from build123d import *

# Parameters (mm, degrees)
F1_DEPTH      = 2.667
F1_DEPTH_BACK = 2.667
F2_W          = 95.25
F2_H          = 4.826
F3_DEPTH      = 9.525
F3_DEPTH_BACK = 9.525
F4_R          = 3.175
F4_R_2        = 7.14375
F5_DEPTH      = 3.556
F6_R          = 1.524
F7_DEPTH      = 10.16


with BuildPart() as f1:
    # F0 (on Right) → F1 (new body, two sides)
    with BuildSketch(Plane.YZ) as f1_sk:
        with BuildLine():
            Line((89.8299359697, 89.8299359697), (0, 0))
            Line((0, 0), (7.6651280605, 0))
            Line((7.6651280605, 0), (95.25, 0))
            Line((95.25, 0), (95.25, 87.5848719395))
            ThreePointArc((95.25, 87.5848719395), (93.2900198978, 90.5181894552), (89.8299359697, 89.8299359697))
        make_face()
        with BuildLine():
            ThreePointArc((38.3256403027, 12.7), (35.3923227869, 14.6599801022), (36.0805762724, 18.1200640303))
            Line((36.0805762724, 18.1200640303), (77.1299359697, 59.1694237276))
            ThreePointArc((77.1299359697, 59.1694237276), (80.5900198978, 59.8576772131), (82.55, 56.9243596973))
            Line((82.55, 56.9243596973), (82.55, 15.875))
            ThreePointArc((82.55, 15.875), (81.6200640303, 13.6299359697), (79.375, 12.7))
            Line((79.375, 12.7), (38.3256403027, 12.7))
        make_face(mode=Mode.SUBTRACT)
    extrude(amount=F1_DEPTH)
    extrude(f1_sk.sketch, amount=-F1_DEPTH_BACK)

    # F2 (on Right) → F3 (join, two sides)
    with BuildSketch(Plane.YZ) as f3_sk:
        with Locations((47.625, -2.413)):
            Rectangle(F2_W, F2_H)
    extrude(amount=F3_DEPTH)
    extrude(f3_sk.sketch, amount=-F3_DEPTH_BACK)

    # F4 (on face) → F5 (cut)
    with BuildSketch(Plane(origin=(0, 0, -4.826), x_dir=(1, 0, 0), z_dir=(0, 0, -1))):
        with Locations((0, -85.09)):
            Circle(F4_R)
        with Locations((0, -10.16)):
            Circle(F4_R)
        with Locations((0, -73.66)):
            Circle(F4_R_2)
        with Locations((0, -21.59)):
            Circle(F4_R_2)
    extrude(amount=-F5_DEPTH, mode=Mode.SUBTRACT)

    # F6 (on face) → F7 (cut)
    with BuildSketch(Plane(origin=(0, 0, -4.826), x_dir=(1, 0, 0), z_dir=(0, 0, -1))):
        with Locations((0, -85.09)):
            Circle(F6_R)
        with Locations((0, -10.16)):
            Circle(F6_R)
    extrude(amount=-F7_DEPTH, mode=Mode.SUBTRACT)


solid = f1.part
Input: part model. Units: mm. Frame: model coordinates. A direction names the side the tool comes from. Coordinates: 2 decimals unless noted, no trailing zeros. Loops run counter-clockwise (first coordinate to the right, second up) from the corner with the lowest first, then second, coordinate; pieces in that order, holes last.
Q1. Contact query for flat-ended pins moving along their axis: pin 1 (5 mm diameter, centred on x = 0, y = 10.16, fed in from -Z); pin 2 (12 mm diameter, centred on y = 12, z = 17, fed in from +X); pin 3 (1.5 mm diameter, centred on x = -1, z = 53, fed in from -Y). Output: stop coordinate, or through.
Q2. Cut plane A-A (z = 22). Output: boundary loops of the cut face in (x, y), then the cut area to 3 significant figures.
Q3. Draft query along Y for faces 6 (the face through (0.04, 56.32, 38.36)), 7 (the face through (0.037, 93.338, 90.498)), 8 (the face through (0, 82.55, 37)), 9 (the face through (-6, 47, 0)). Return one class per face: +Y half, -Y half, draft (parallel to the pull), parting line (faces both ways), or undercut.
Q4. Material intervals for line 1 (Y direction, x = 0, z = -3.2) (3 decimals); line 2 (X direction, y = 21.59, z = -2.5) (3 decimals); line 3 (Z direction, x = -3.75, y = 45.5), sorted ascending.
Q5. Cut plane D-D (y = 63). Output: boundary loops of the cut face in (x, z) (3 decimals), then the cut area to 3 significant figures.
Q6. Cut plane B-B (y = 34). Output: boundary loops of the cut face in (x, z) (3 decimals).
Q7. Set-up query: faces 1 (the face through (0, 46, 46)), 2 (the face through (0.04, 80.54, 59.88)), 3 (the face through (-2.667, 54, 39)), 4 (the face through (0, 21, -1.27)), 5 (the face through (9.525, 47, -2)). Return all of +Z, -Z, +X, -X, +Y, -Y with unobstructed straight access to the full face (end or side cutting, diameter ignored); none if empty.
Q8. Cut plane C-C (x = -4.75). Output: boundary loops of the cut face in (y, z).
Working result:
1. pin 1: stops at z = -1.27
1. pin 2: stops at x = 2.67
1. pin 3: stops at y = 52.25
2. outline: (-2.67, 22) - (2.67, 22) - (2.67, 39.96) - (-2.67, 39.96) - close; (-2.67, 82.55) - (2.67, 82.55) - (2.67, 95.25) - (-2.67, 95.25) - close
2. area: 164 mm2
3. face 6: undercut
3. face 7: parting line
3. face 8: undercut
3. face 9: draft
4. line 1: y = 0 to 6.985, 13.335 to 14.446, 28.734 to 66.516, 80.804 to 81.915, 88.265 to 95.25
4. line 2: x = -9.525 to -7.144, 7.144 to 9.525
4. line 3: z = -4.83 to 0
5. outline: (-9.525, -4.826) - (9.525, -4.826) - (9.525, 0) - (2.667, 0) - (2.667, 12.7) - (-2.667, 12.7) - (-2.667, 0) - (-9.525, 0) - close; (-2.667, 45.039) - (2.667, 45.039) - (2.667, 63) - (-2.667, 63) - close
5. area: 255 mm2
6. outline: (-9.525, -4.826) - (9.525, -4.826) - (9.525, 0) - (2.667, 0) - (2.667, 34) - (-2.667, 34) - (-2.667, 0) - (-9.525, 0) - close
7. face 1: +Z, +X, -X, -Y
7. face 2: +X, -X
7. face 3: +Z, -X, +Y, -Y
7. face 4: -Z
7. face 5: +Z, -Z, +X, +Y, -Y
8. outline: (0, -4.83) - (16.25, -4.83) - (16.25, -1.27) - (26.93, -1.27) - (26.93, -4.83) - (68.32, -4.83) - (68.32, -1.27) - (79, -1.27) - (79, -4.83) - (95.25, -4.83) - (95.25, 0) - (0, 0) - close
